The listing builds one solid part. Answer for the finished solid, in the listing's coordinates (mm). Give positions to 0.01 mm unless a question says otherwise; leave off trailing zeros. Write each loop counter-clockwise with the first axis right and the second up, starting at its lowest first coordinate (ties: lowest second). Pieces come first, ordered by that corner, then holes. Notation, with made-up numbers: M 43.5,53 L 90.5,53 A9 cw 90.5,69 Z; hole C 2,7.5 d9. An arc over 180 degrees is marked long. Return JSON: item names as keys, results as strings.
Autodesk Inventor part; units mm, degrees
ref_plane "YZ Plane" through (0, 0, 0) normal (1, 0, 0) x (0, 1, 0)
ref_plane "XZ Plane" through (0, 0, 0) normal (0, 1, 0) x (-1, 0, 0)
ref_plane "XY Plane" through (0, 0, 0) normal (0, 0, 1) x (1, 0, 0)
sketch "Sketch1" plane through (0, 0, 0) normal (0, 0, 1) x (1, 0, 0)
  line L0 (-100, -10) -> (100, -10)
  line L1 (100, -10) -> (100, 10)
  line L2 (100, 10) -> (-100, 10)
  line L3 (-100, 10) -> (-100, -10)
  line L4 (-100, -10) -> (100, 10) construction
  line L5 (100, -10) -> (-100, 10) construction
  point P0 (0, 0)
  dimension "d0" = 200
  dimension "d1" = 20
extrude "Extrusion1" add sketch "Sketch1" along normal blind 3
sketch "Sketch2" plane through (0, 0, 3) normal (0, 0, 1) x (1, 0, 0)
  circle A0 centre (-90, 0) radius 3
  line L0 (-100, 10) -> (-100, -10)
  line L1 (100, 10) -> (-100, 10)
  point P0 (0, 0)
  dimension "d5" = 6
  dimension "d6" = 10
  dimension "d7" = 10
extrude "Extrusion2" cut sketch "Sketch2" against normal blind 3
pattern_linear "Rectangular Pattern1" count 10 spacing 20 along (1, 0, 0) of "Extrusion2"
fillet "Fillet1" radius 2 4 edges at (100, 10, 1.5) (100, -10, 1.5) (-100, -10, 1.5) (-100, 10, 1.5)
properties part number "Noi nhom 20100"
Item 1: Determine the mould class of faces 1 (the cylindrical face through (-12.4, -1.8, 1.5)), 2 (the flat face through (-1, 0, 3)) for opening direction X: +X half, -X half, draft (parallel to the pull), parting line (faces both ways), or undercut.
Geometry results:
{"face 1": "undercut", "face 2": "draft"}
Item 2: A cutting plane is placed at A-A, the plane x = -70. Write down the section's boundary in (y, z), plus the area to 3 significant figures.
Geometry results:
{"outline": "M -10,0 L -3,0 L -3,3 L -10,3 Z; M 3,0 L 10,0 L 10,3 L 3,3 Z", "area": "42.0 mm2"}
Item 3: A cutting plane is placed at B-B, the plane z = 2.3. Count the separate pieces of the cut face and the enclosed holes in it, plus the area to 3 significant figures.
Geometry results:
{"separate pieces": "1", "enclosed holes": "10", "area": "3,710 mm2"}
Item 4: Find the intervals of material crossed by line 1 (Y direction, x = -70, z = 2.4); line 2 (Y direction, x = -72, z = 1.9), in increasing order.
Geometry results:
{"line 1": "y = -10 to -3, 3 to 10", "line 2": "y = -10 to -2.24, 2.24 to 10"}
